The drawing under review shows one solid part. Ordinate dimensions are in mm from its lowest x, y, z. Coordinates: 2 decimals unless noted, no trailing zeros. Loops run counter-clockwise (first coordinate to the right, second up) from the corner with the lowest first, then second, coordinate; pieces in that order, holes last. Notation, with made-up numbers: M 51,31.5 L 110,31.5 A31 ccw 110,67.5 Z; hole C -15,62 d4. An arc over 180 degrees is marked long. Answer as a JSON object with one key per item and string values. Group by question number.
1. Consider section B-B (x = 765.5). State the section outline as (y, z) points, then the cut area to 3 significant figures.
2. Insertion check: pin 1 (12 mm diameter, centred on x = 133.5, y = 111, fed in from -Z). The pin has a flat end and moves straight along its axis. Give the tip position at first contact, or say it passes through.
3. Consider section A-A (y = 311). State the section outline as (x, z) points, then the cut area to 3 significant figures.
4. To check wall thickness, follow probe 1 along Z at (x, y) = (250, 20.5). State the ranges of the line that lie inside material, in increasing order.
5. Consider section C-C (z = 377). Count the separate pieces of the cut face and the enclosed holes in it, then the cut area to 3 significant figures.
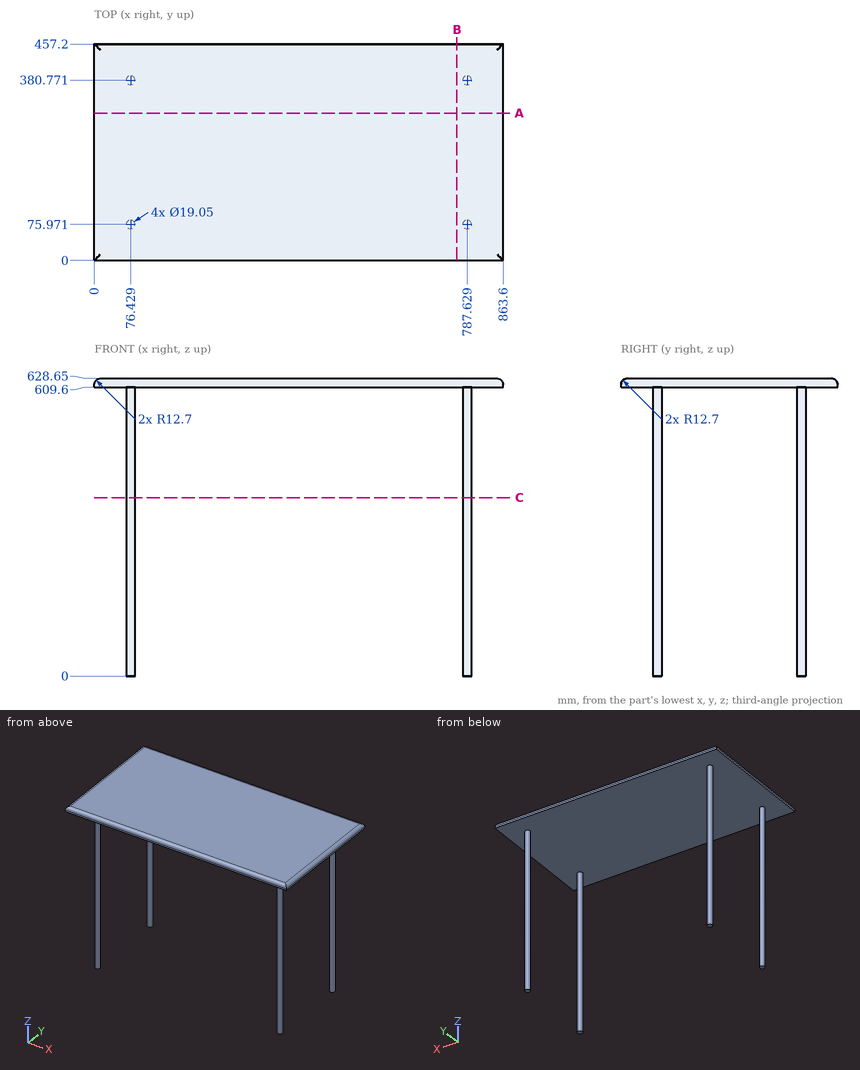
Findings below:
{
 "1": {"outline": "M 0,609.6 L 457.2,609.6 L 457.2,615.95 A12.7 ccw 444.5,628.65 L 12.7,628.65 A12.7 ccw 0,615.95 Z", "area": "8,640 mm^2"},
 "2": {"pin 1": "stops at z = 609.6"},
 "3": {"outline": "M 0,609.6 L 863.6,609.6 L 863.6,615.95 A12.7 ccw 850.9,628.65 L 12.7,628.65 A12.7 ccw 0,615.95 Z", "area": "16,400 mm^2"},
 "4": {"probe 1": "z = 609.6 to 628.65"},
 "5": {"separate pieces": "4", "enclosed holes": "0", "area": "1,140 mm^2"}
}
